```python
from build123d import *

# Parameters (mm, degrees)
SKETCH1_R           = 11
SKETCH1_R_2         = 7.7
BOSS_EXTRUDE1_DEPTH = 30
BOSS_EXTRUDE2_START = 30
SKETCH1_2_R         = 11
SKETCH1_2_R_2       = 7.7
BOSS_EXTRUDE2_DEPTH = 5
BOSS_EXTRUDE3_START = 35
SKETCH1_4_R         = 11
SKETCH1_4_R_2       = 7.7
SKETCH1_4_R_3       = 3.15
BOSS_EXTRUDE3_DEPTH = 15
SKETCH1_5_R         = 12.5
SKETCH1_5_R_2       = 11
BOSS_EXTRUDE4_DEPTH = 30
SKETCH2_R           = 1.85
CUT_EXTRUDE1_DEPTH  = 58.282196187
SKETCH2_7_R         = 2.371596242
CUT_EXTRUDE2_DEPTH  = 4
SKETCH2_8_R         = 2.371596242
CUT_EXTRUDE3_DEPTH  = 58.282196274
FILLET1_R           = 7
FILLET2_R           = 2
CHAMFER1_SIZE       = 3


with BuildPart() as part:
    # Sketch1 → Boss-Extrude1 (new body)
    with BuildSketch(Plane(origin=(0, 0, 0), x_dir=(1, 0, 0), z_dir=(0, 1, 0))):
        with Locations(Location((0, 0, 0), (0, 0, 270))):
            Circle(SKETCH1_R)
        with Locations(Location((0, 0, 0), (0, 0, 270))):
            Circle(SKETCH1_R_2, mode=Mode.SUBTRACT)
    extrude(amount=BOSS_EXTRUDE1_DEPTH)

    # Sketch1<2> → Boss-Extrude2 (add)
    # profile 1 of 6: a face of its own
    with BuildSketch(Plane(origin=(0, 0, 0), x_dir=(1, 0, 0), z_dir=(0, 1, 0)).offset(BOSS_EXTRUDE2_START)):
        with Locations(Location((0, 0, 0), (0, 0, 270))):
            Circle(SKETCH1_2_R)
        with Locations(Location((0, 0, 0), (0, 0, 270))):
            Circle(SKETCH1_2_R_2, mode=Mode.SUBTRACT)
    # profile 2 of 6: a face of its own
    with BuildSketch(Plane(origin=(0, 0, 0), x_dir=(1, 0, 0), z_dir=(0, 1, 0)).offset(BOSS_EXTRUDE2_START)):
        with Locations(Location((0, 0, 0), (0, 0, 270))):
            Circle(SKETCH1_2_R_2)
    # profile 3 of 6: a face of its own
    with BuildSketch(Plane(origin=(0, 0, 0), x_dir=(1, 0, 0), z_dir=(0, 1, 0)).offset(BOSS_EXTRUDE2_START)):
        with BuildLine():
            ThreePointArc((2, 2.433618705), (0, 3.15), (-2, 2.433618705))
            Line((-2, 2.433618705), (2, 2.433618705))
        make_face()
    # profile 4 of 6: a face of its own
    with BuildSketch(Plane(origin=(0, 0, 0), x_dir=(1, 0, 0), z_dir=(0, 1, 0)).offset(BOSS_EXTRUDE2_START)):
        with BuildLine():
            Line((2, 2.433618705), (-2, 2.433618705))
            ThreePointArc((-2, 2.433618705), (-1.345826883, -2.848025632), (3.15, 0))
            ThreePointArc((3.15, 0), (2.848025632, 1.345826883), (2, 2.433618705))
        make_face()
    # profile 5 of 6: a face of its own
    with BuildSketch(Plane(origin=(0, 0, 0), x_dir=(1, 0, 0), z_dir=(0, 1, 0)).offset(BOSS_EXTRUDE2_START)):
        with BuildLine():
            ThreePointArc((2, 2.433618705), (0, 3.15), (-2, 2.433618705))
            Line((-2, 2.433618705), (2, 2.433618705))
        make_face()
    # profile 6 of 6: a face of its own
    with BuildSketch(Plane(origin=(0, 0, 0), x_dir=(1, 0, 0), z_dir=(0, 1, 0)).offset(BOSS_EXTRUDE2_START)):
        with BuildLine():
            Line((2, 2.433618705), (-2, 2.433618705))
            ThreePointArc((-2, 2.433618705), (-1.345826883, -2.848025632), (3.15, 0))
            ThreePointArc((3.15, 0), (2.848025632, 1.345826883), (2, 2.433618705))
        make_face()
    extrude(amount=BOSS_EXTRUDE2_DEPTH)

    # Sketch1<4> → Boss-Extrude3 (add)
    # profile 1 of 3: a face of its own
    with BuildSketch(Plane(origin=(0, 0, 0), x_dir=(1, 0, 0), z_dir=(0, 1, 0)).offset(BOSS_EXTRUDE3_START)):
        with Locations(Location((0, 0, 0), (0, 0, 270))):
            Circle(SKETCH1_4_R)
        with Locations(Location((0, 0, 0), (0, 0, 270))):
            Circle(SKETCH1_4_R_2, mode=Mode.SUBTRACT)
    # profile 2 of 3: a face of its own
    with BuildSketch(Plane(origin=(0, 0, 0), x_dir=(1, 0, 0), z_dir=(0, 1, 0)).offset(BOSS_EXTRUDE3_START)):
        with Locations(Location((0, 0, 0), (0, 0, 270))):
            Circle(SKETCH1_4_R_2)
        Circle(SKETCH1_4_R_3, mode=Mode.SUBTRACT)
    # profile 3 of 3: a face of its own
    with BuildSketch(Plane(origin=(0, 0, 0), x_dir=(1, 0, 0), z_dir=(0, 1, 0)).offset(BOSS_EXTRUDE3_START)):
        with BuildLine():
            ThreePointArc((2, 2.433618705), (0, 3.15), (-2, 2.433618705))
            Line((-2, 2.433618705), (2, 2.433618705))
        make_face()
    extrude(amount=BOSS_EXTRUDE3_DEPTH)

    # Sketch1<5> → Boss-Extrude4 (add)
    with BuildSketch(Plane(origin=(0, 0, 0), x_dir=(1, 0, 0), z_dir=(0, 1, 0))):
        with Locations(Location((0, 0, 0), (0, 0, 270))):
            Circle(SKETCH1_5_R)
        with Locations(Location((0, 0, 0), (0, 0, 270))):
            Circle(SKETCH1_5_R_2, mode=Mode.SUBTRACT)
    extrude(amount=BOSS_EXTRUDE4_DEPTH)

    # Sketch2 → Cut-Extrude1 (cut, through all)
    with BuildSketch(Plane(origin=(0, 0, -12.5), x_dir=(-1, 0, 0), z_dir=(0, 0, -1))):
        with Locations(Location((0, 43.042161893, 0), (0, 0, 90))):
            Circle(SKETCH2_R)
    extrude(amount=-CUT_EXTRUDE1_DEPTH, mode=Mode.SUBTRACT)

    # Sketch2<7> → Cut-Extrude2 (cut)
    # profile 1 of 2: a face of its own
    with BuildSketch(Plane(origin=(0, 0, -12.5), x_dir=(-1, 0, 0), z_dir=(0, 0, -1))):
        Polygon((-2.107328483, 11.35), (2.107328483, 11.35), (4.214656965, 15), (2.107328483, 18.65), (-2.107328483, 18.65), (-4.214656965, 15), align=None)
        with Locations((0, 15)):
            Circle(SKETCH2_7_R, mode=Mode.SUBTRACT)
    # profile 2 of 2: a face of its own
    with BuildSketch(Plane(origin=(0, 0, -12.5), x_dir=(-1, 0, 0), z_dir=(0, 0, -1))):
        with Locations((0, 15)):
            Circle(SKETCH2_7_R)
    extrude(amount=-CUT_EXTRUDE2_DEPTH, mode=Mode.SUBTRACT)

    # Sketch2<8> → Cut-Extrude3 (cut, through all)
    with BuildSketch(Plane(origin=(0, 0, -12.5), x_dir=(-1, 0, 0), z_dir=(0, 0, -1))):
        with Locations((0, 15)):
            Circle(SKETCH2_8_R)
    extrude(amount=-CUT_EXTRUDE3_DEPTH, mode=Mode.SUBTRACT)

    # Fillet1
    # the kernel refuses this fillet: 7 mm, written as the material it takes off along each edge
    with BuildSketch(Plane(origin=(0, 30, 0), x_dir=(0, 0, 1), z_dir=(-1, 0, 0))) as fillet1_piece_1:
        with BuildLine():
            CenterArc((5.5, -4.330127019), FILLET1_R, 0, 38.213210702)
            Line((12.5, -4.330127019), (12.64, -4.330127019))
            Line((12.64, -4.330127019), (12.64, 0))
            Line((12.64, 0), (12.5, 0.14))
            ThreePointArc((12.5, 0.14), (11.75, 0.14), (11.11, 0.08660254))
            Line((11.11, 0.08660254), (11, 0))
        make_face()
    revolve(axis=Axis((0, 30, 0), (0, 1, 0)), mode=Mode.SUBTRACT)

    # Fillet2
    fillet2_edges = [part.edges().sort_by_distance(p)[0] for p in [
        (0, 0, -12.5),
        (0, 0, -7.7),
    ]]
    fillet(fillet2_edges, radius=FILLET2_R)

    # Chamfer1
    chamfer1_edges = [part.edges().sort_by_distance(p)[0] for p in [
        (0, 50, -11),
    ]]
    chamfer(chamfer1_edges, length=CHAMFER1_SIZE)


solid = part.part
```
The model under review builds one solid part; all positions refer to its coordinate system, in mm. A direction names the side the tool comes from. Round coordinates to 2 decimals unless told otherwise and drop trailing zeros. Write each loop counter-clockwise with the first axis right and the second up, starting at its lowest first coordinate (ties: lowest second). Pieces come first, ordered by that corner, then holes. Notation, with made-up numbers: (10, 54.25) - (34, 54.25) arc R27 ccw to (34, 83.25) - close; hole circle Ø5 at (75, 11). An arc over 180 degrees is marked (long way). One line per question, with ' | ' between items.
Item 1: To check wall thickness, follow probe 1 along Y at (x, z) = (0, -7.6); probe 2 along Y at (x, z) = (0, 10.45); probe 3 along X at (y, z) = (39, 0). State the ranges of each line that lie inside material, in increasing order.
Resolved:
probe 1: y = 30 to 41.19, 44.89 to 50 | probe 2: y = 0 to 12.63, 17.37 to 41.19, 44.89 to 47.55 | probe 3: x = -11 to -3.15, 3.15 to 11
Item 2: The part is to be moulded in two halves that separate along Z. For faces 1 (the face through (0, 35, 0)), 2 (the face through (-3.176, 16.799, -10.437)), 3 (the face through (-7.952, 49.854, -1.766)), say which applies: pulls with the +Z half, pulls with the -Z half, needs draft (parallel to the pull), parting line crosses it, or undercut.
Resolved:
face 1: undercut | face 2: needs draft | face 3: parting line crosses it
Item 3: Add section C-C, the plane y = 4.5. Give the boundary of the cut face in (x, z), then the cut area to 3 significant figures.
Resolved:
outline: circle Ø25 at (0, 0); hole circle Ø15.4 at (0, 0) | area: 305 mm2
Item 4: For faces 4 (the face through (-4.213, 38.381, 10.161)), 5 (the face through (0, 11.35, -11)), 6 (the face through (-2.949, 15.804, 7.113)), list the 3-axis set-ups (+Z, -Z, +X, -X, +Y, -Y) from which the entire face can be reached by the end or side of a thin tool; tool diameter is ignored.
Resolved:
face 4: +Y | face 5: -Z | face 6: -Y
Item 5: For P1, Ø10, axis at y = 31, z = 6.5, coming from the +X side; P2, Ø4.5, axis at x = 2, z = 3, coming from the -Y side; P3, Ø1, axis at y = 26.5, z = -6.5, coming from the -X side, all flat-tipped, find the tip position at first contact; note any pin that passes through.
Resolved:
P1: stops at x = 11.9 | P2: stops at y = 30 | P3: stops at x = -10.92
Item 6: Add section B-B, the plane y = 33.5. Give the boundary of the cut face in (x, z), then the cut area to 3 significant figures.
Resolved:
outline: circle Ø22 at (0, 0) | area: 380 mm2
Item 7: Add section A-A, the plane x = 0. State how many separate pieces and enclosed holes the cut face has, then the cut area to 3 significant figures.
Resolved:
separate pieces: 5 | enclosed holes: 0 | area: 511 mm2
